Part print with two shaded views. Sizes in mm from the minimum x, y, z corner. Round coordinates to 2 decimals unless told otherwise and drop trailing zeros. Order: outer loops, then holes, each group sorted by start corner. A loop starts at its lowest first (then second) coordinate and runs counter-clockwise, first axis right, second up. Notation, with made-up numbers: M -6,-30.75 L 37,-30.75 A21 ccw 37,3.25 Z; hole C -31,13 d5. An arc over 180 degrees is marked long. One line per question, with ' | ' between items. Start each with the question number.
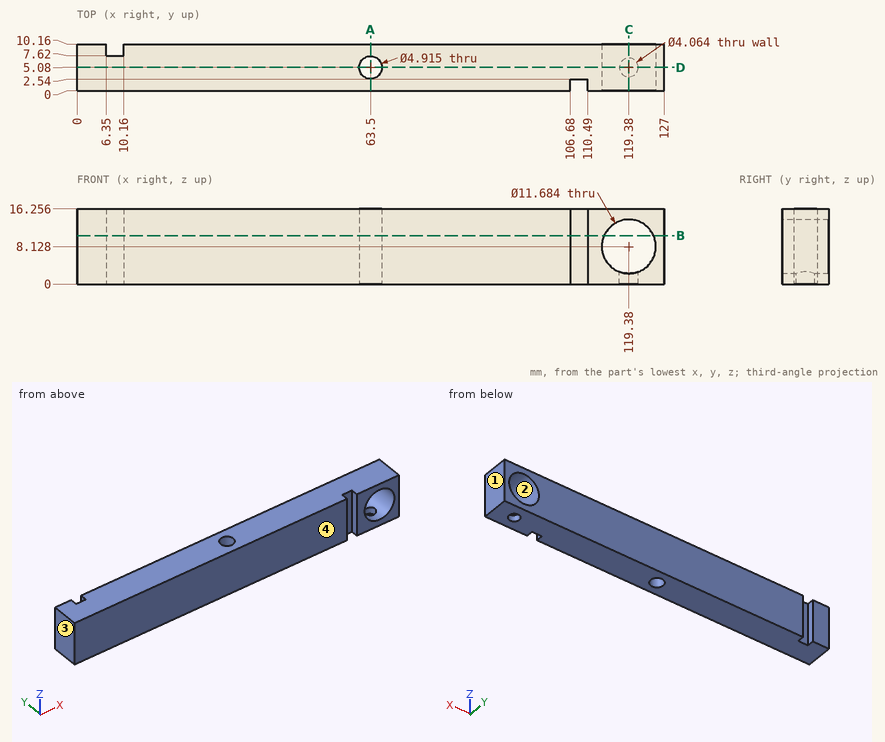
Item 1: Cut at C-C on x = 119.38. Write the cut outline in (y, z).
Item 2: Two-plate mould, pull along X, no slides. Class the marked faces 1, 2, 3 and 4: +X half, -X half, draft (parallel to the pull), parting line (faces both ways), or undercut.
Item 3: Cut at D-D on y = 5.08. Write the cut outline in (x, z), then the cut area to 3 significant figures.
Item 4: Cut at B-B on z = 10.5. Count the separate pieces of the cut face and the enclosed holes in it, then the cut area to 3 significant figures.
Item 5: Flat gauge pins, fed straight in: pin 1 (1.3 mm diameter, centred on y = 1, z = 7, fed in from -X); pin 2 (3.5 mm diameter, centred on x = 119.38, y = 5.08, fed in from -Z); pin 3 (3 mm diameter, centred on x = 8, z = 5, fed in from +Y); pin 4 (4.5 mm diameter, centred on x = 63.5, y = 5.08, fed in from -Z). Where does each tip first touch, or does it go through?
Item 6: Wall check: line 1 along Y through (x, z) = (119.38, 0.5); line 2 along X through (y, z) = (5, 14.75); line 3 along Y through (x, z) = (63.5, 9). Give the ranges that are in metal, low to high. Write a range as [from, to].
Item 7: Cut at A-A on x = 63.5. Write the cut outline in (y, z).
Results found:
1) outline: M 0,0 L 3.05,0 L 3.05,2.29 L 0,2.29 Z; M 0,13.97 L 10.16,13.97 L 10.16,16.26 L 0,16.26 Z; M 7.11,0 L 10.16,0 L 10.16,2.29 L 7.11,2.29 Z
2) face 1: +X half | face 2: undercut | face 3: -X half | face 4: draft
3) outline: M 0,0 L 61.04,0 L 61.04,16.26 L 0,16.26 Z; M 65.96,0 L 117.35,0 L 117.35,2.65 A5.84 cw long 121.41,2.65 L 121.41,0 L 127,0 L 127,16.26 L 65.96,16.26 Z | area: 1,870 mm^2
4) separate pieces: 2 | enclosed holes: 1 | area: 1,140 mm^2
5) pin 1: stops at x = 0 | pin 2: stops at z = 13.7 | pin 3: stops at y = 7.62 | pin 4: passes through
6) line 1: y = [0, 3.05], [7.11, 10.16] | line 2: x = [0, 61.04], [65.96, 127] | line 3: y = [0, 2.62], [7.54, 10.16]
7) outline: M 0,0 L 2.62,0 L 2.62,16.26 L 0,16.26 Z; M 7.54,0 L 10.16,0 L 10.16,16.26 L 7.54,16.26 Z
